```python
from build123d import *

# Parameters (mm, degrees)
SKETCH11_W         = 485.793761844
SKETCH11_H         = 595.960227968
CUT_EXTRUDE1_DEPTH = 130.789538956


with BuildPart() as part:
    # Sweep-Thin1: sweep along a path in Sketch2
    with BuildLine(Plane(origin=(0, 0, 0), x_dir=(1, 0, 0), z_dir=(0, 1, 0))) as sweep_thin1_path:
        Line((0, 169.789538956), (0, 157.289538956))
        Line((0, 157.289538956), (0, 30))
        ThreePointArc((0, 30), (-8.786796564, 8.786796564), (-30, 0))
        Line((-30, 0), (-200, 0))
        ThreePointArc((-200, 0), (-221.213203436, 8.786796564), (-230, 30))
        Line((-230, 30), (-230, 40))
    # Sketch6 → Sweep-Thin1 (sweep)
    with BuildSketch(Plane.XY.offset(-40)):
        with BuildLine():
            Line((-225.5, 12.5), (-234.5, 12.5))
            ThreePointArc((-234.5, 12.5), (-240.156854249, 10.156854249), (-242.5, 4.5))
            Line((-242.5, 4.5), (-242.5, -4.5))
            ThreePointArc((-242.5, -4.5), (-240.156854249, -10.156854249), (-234.5, -12.5))
            Line((-234.5, -12.5), (-225.5, -12.5))
            ThreePointArc((-225.5, -12.5), (-219.843145751, -10.156854249), (-217.5, -4.5))
            Line((-217.5, -4.5), (-217.5, 4.5))
            ThreePointArc((-217.5, 4.5), (-219.843145751, 10.156854249), (-225.5, 12.5))
        make_face()
        with BuildLine():
            Line((-225.5, 9.5), (-234.5, 9.5))
            ThreePointArc((-234.5, 9.5), (-238.035533906, 8.035533906), (-239.5, 4.5))
            Line((-239.5, 4.5), (-239.5, -4.5))
            ThreePointArc((-239.5, -4.5), (-238.035533906, -8.035533906), (-234.5, -9.5))
            Line((-234.5, -9.5), (-225.5, -9.5))
            ThreePointArc((-225.5, -9.5), (-221.964466094, -8.035533906), (-220.5, -4.5))
            Line((-220.5, -4.5), (-220.5, 4.5))
            ThreePointArc((-220.5, 4.5), (-221.964466094, 8.035533906), (-225.5, 9.5))
        make_face(mode=Mode.SUBTRACT)
    sweep(path=sweep_thin1_path.line)

    # Sketch11 → Cut-Extrude1 (cut, through all)
    with BuildSketch(Plane.XY.offset(-40)):
        with Locations((212.093031721, 3.359547151)):
            Rectangle(SKETCH11_W, SKETCH11_H)
    extrude(amount=-CUT_EXTRUDE1_DEPTH, mode=Mode.SUBTRACT)


solid = part.part
```
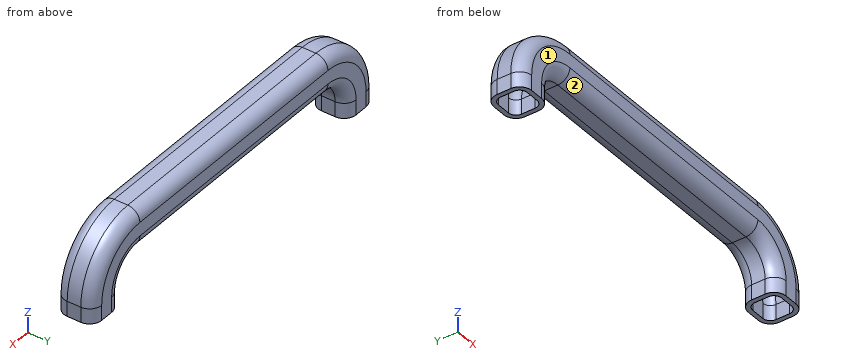
Verification items for the finished model (mm, model axes). Face numbers are marked on the shaded views. Give positions to 0.01 mm unless a question says otherwise; leave off trailing zeros. Loops run counter-clockwise (first coordinate to the right, second up) from the corner with the lowest first, then second, coordinate; pieces in that order, holes last.
1. Mould release check, pull along X, two halves, no side actions. Record for the marked faces 1 and 2: released by +X, released by -X, zero draft, split by the parting line, or undercut.
2. Thickness scan on line 1 (X direction, y = -4.5, z = -33.5); line 2 (Z direction, x = -166, y = -2.75); line 3 (Y direction, x = -70.5, z = -5). Record the ranges inside material, lowest first.
3. Go/stop test with flat-tipped pins: pin 1 Ø10 at (x, y) = (-135, -2) entering from -Z; pin 2 Ø12 at (y, z) = (7, -16) entering from -X; pin 3 Ø1.5 at (x, z) = (-126.5, -14.5) entering from -Y; pin 4 Ø2 at (y, z) = (-9.5, 3) entering from -X. Record where each tip stops, or that it passes through.
4. Section check C-C, the plane x = -109. Enter the section's corners in (y, z).
5. Section check A-A, the plane y = -0.75. Enter the section's corners in (x, z).
6. Section check B-B, the plane z = -33.5. Count the separate pieces of the cut face and the enclosed holes in it, then the cut area to 3 significant figures.
Geometry says:
1. face 1: zero draft
1. face 2: undercut
2. line 1: x = -242.5 to -239.5, -220.5 to -217.5, -12.5 to -9.5, 9.5 to 12.5
2. line 2: z = -12.5 to -9.5, 9.5 to 12.5
2. line 3: y = -12.48 to -9.47, 9.47 to 12.48
3. pin 1: stops at z = -12.5
3. pin 2: stops at x = -241.66
3. pin 3: passes through
3. pin 4: stops at x = -225.67
4. outline: (-12.5, -4.5) arc R8 ccw to (-4.5, -12.5) - (4.5, -12.5) arc R8 ccw to (12.5, -4.5) - (12.5, 4.5) arc R8 ccw to (4.5, 12.5) - (-4.5, 12.5) arc R8 ccw to (-12.5, 4.5) - close; hole (-9.5, -4.5) arc R5 ccw to (-4.5, -9.5) - (4.5, -9.5) arc R5 ccw to (9.5, -4.5) - (9.5, 4.5) arc R5 ccw to (4.5, 9.5) - (-4.5, 9.5) arc R5 ccw to (-9.5, 4.5) - close
5. outline: (-242.5, -40) - (-239.5, -40) - (-239.5, -30) arc R39.5 cw to (-200, 9.5) - (-30, 9.5) arc R39.5 cw to (9.5, -30) - (9.5, -40) - (12.5, -40) - (12.5, -30) arc R42.5 ccw to (-30, 12.5) - (-200, 12.5) arc R42.5 ccw to (-242.5, -30) - close; (-220.5, -40) - (-217.5, -40) - (-217.5, -30) arc R17.5 cw to (-200, -12.5) - (-30, -12.5) arc R17.5 cw to (-12.5, -30) - (-12.5, -40) - (-9.5, -40) - (-9.5, -30) arc R20.5 ccw to (-30, -9.5) - (-200, -9.5) arc R20.5 ccw to (-220.5, -30) - close
6. separate pieces: 2
6. enclosed holes: 2
6. area: 461 mm2
